from build123d import *

# Parameters (mm, degrees)
EXTRUDE1_DEPTH     = 17.78
SKETCH4_R          = 3.175000003
SKETCH4_R_2        = 3.175000002
CUT_EXTRUDE1_DEPTH = 17.78
SKETCH6_R          = 1.5875
SKETCH6_R_2        = 1.587500002
SKETCH6_R_3        = 2.777849083
CUT_EXTRUDE3_DEPTH = 17.78
SKETCH5_W          = 17.78
SKETCH5_H          = 63.50740041
SKETCH5_H_2        = 63.507400408
CUT_EXTRUDE2_DEPTH = 5.08
SKETCH7_R          = 3.302
SKETCH7_R_2        = 3.302000002
CUT_EXTRUDE4_DEPTH = 5.08
SKETCH9_R          = 3.175
CUT_EXTRUDE5_DEPTH = 17.78


with BuildPart() as part:
    # Sketch3 → Extrude1 (new body)
    with BuildSketch(Plane.XY):
        Polygon((10806.641666666, -6342.0625), (11409.891666666, -6342.0625), (11409.891666666, -5818.736838581), (11378.141666665, -5818.736838581), (11378.141666665, -5742.536838581), (10838.391666667, -5742.536838581), (10838.391666667, -5818.736838581), (10806.641666666, -5818.736838581), align=None)
    extrude(amount=-EXTRUDE1_DEPTH)

    # Sketch4 → Cut-Extrude1 (cut)
    with BuildSketch(Plane.XY):
        with Locations((11380.386730695, -5816.491774551)):
            Circle(SKETCH4_R)
        with Locations((10836.146602637, -5816.491774551)):
            Circle(SKETCH4_R_2)
    extrude(amount=-CUT_EXTRUDE1_DEPTH, mode=Mode.SUBTRACT)

    # Sketch6 → Cut-Extrude3 (cut)
    with BuildSketch(Plane.XY):
        with Locations((10851.409166666, -6294.4375)):
            Circle(SKETCH6_R)
        with Locations((10908.241666666, -6326.8225)):
            Circle(SKETCH6_R)
        with Locations((11108.266666666, -6326.8225)):
            Circle(SKETCH6_R)
        with Locations((11308.291666666, -6326.8225)):
            Circle(SKETCH6_R)
        with Locations((11365.124166666, -6294.4375)):
            Circle(SKETCH6_R)
        with Locations((11365.124166666, -6237.2875)):
            Circle(SKETCH6_R)
        with Locations((11333.691666666, -6220.099669291)):
            Circle(SKETCH6_R)
        with Locations((11365.124166666, -6180.1375)):
            Circle(SKETCH6_R)
        with Locations((11333.691666666, -6042.299669291)):
            Circle(SKETCH6_R)
        with Locations((11333.691666666, -5864.499669291)):
            Circle(SKETCH6_R)
        with Locations((11369.251666663, -5793.344238991)):
            Circle(SKETCH6_R_2)
        with Locations((11369.251666663, -5755.236838581)):
            Circle(SKETCH6_R_2)
        with Locations((10847.281666666, -5755.236838581)):
            Circle(SKETCH6_R)
        with Locations((10847.281666666, -5793.344238991)):
            Circle(SKETCH6_R)
        with Locations((10882.841666666, -6042.299669291)):
            Circle(SKETCH6_R_3)
        with Locations((10851.409166666, -6180.1375)):
            Circle(SKETCH6_R)
        with Locations((10882.841666666, -6220.099669291)):
            Circle(SKETCH6_R)
        with Locations((10851.409166666, -6237.2875)):
            Circle(SKETCH6_R)
        with Locations((10882.841666666, -5864.499669291)):
            Circle(SKETCH6_R)
    extrude(amount=-CUT_EXTRUDE3_DEPTH, mode=Mode.SUBTRACT)

    # Sketch5 → Cut-Extrude2 (cut)
    with BuildSketch(Plane.XY):
        Polygon((11108.266666666, -6317.9325), (10806.641666666, -6317.9325), (10806.641666666, -6335.7125), (11409.891666666, -6335.7125), (11409.891666666, -6317.9325), align=None)
        with Locations((10847.281666667, -5774.290538786)):
            Rectangle(SKETCH5_W, SKETCH5_H)
        with Locations((11369.251666665, -5774.290538785)):
            Rectangle(SKETCH5_W, SKETCH5_H_2)
    extrude(amount=-CUT_EXTRUDE2_DEPTH, mode=Mode.SUBTRACT)

    # Sketch7 → Cut-Extrude4 (cut)
    with BuildSketch(Plane.XY):
        with Locations((10853.926602637, -5803.79917496)):
            Circle(SKETCH7_R)
        with Locations((11362.606730695, -5803.799174959)):
            Circle(SKETCH7_R_2)
    extrude(amount=-CUT_EXTRUDE4_DEPTH, mode=Mode.SUBTRACT)

    # Sketch9 → Cut-Extrude5 (cut)
    with BuildSketch(Plane.XY):
        with Locations((10914.541654066, -5760.644320781)):
            Circle(SKETCH9_R)
        with Locations((10971.741666666, -5760.644320781)):
            Circle(SKETCH9_R)
        with Locations((11244.741654066, -5760.644320781)):
            Circle(SKETCH9_R)
        with Locations((11301.941666666, -5760.644320781)):
            Circle(SKETCH9_R)
    extrude(amount=-CUT_EXTRUDE5_DEPTH, mode=Mode.SUBTRACT)


solid = part.part
The listing builds one solid part. Answer for the finished solid, in the listing's coordinates (mm). A direction names the side the tool comes from. Coordinates: 2 decimals unless noted, no trailing zeros. Write each loop counter-clockwise with the first axis right and the second up, starting at its lowest first coordinate (ties: lowest second). Pieces come first, ordered by that corner, then holes. Notation, with made-up numbers: M 45,39.5 L 76,39.5 A26 ccw 76,66.5 Z; hole C 52.25,-7 d1. An arc over 180 degrees is marked long. Write each question's results on one line, items separated by ' | '.
Item 1: Which of the six approach directions +Z, -Z, +X, -X, +Y, -Y give full straight-line access (tool end or side, diameter ignored) to faces 1 (the face through (11396, -5818.737, -9)), 2 (the face through (11104, -6038, -17.78)), 3 (the face through (10820, -5818.737, -9))?
Answer below:
face 1: +Z, -Z, +X, +Y | face 2: -Z, +X, -X, +Y, -Y | face 3: +Z, -Z, -X, +Y
Item 2: Consider probe 1 along Y at (x, z) = (10983.5, -1.5); probe 2 along X at (y, z) = (-5807, -13.75); probe 3 along X at (y, z) = (-5778.5, -3.75). Determine where each line is inside the solid, lowest interval first. Write a range as [from, to].
Answer below:
probe 1: [-6342.06, -6335.71], [-6317.93, -5742.54] | probe 2: [10838.39, 11378.14] | probe 3: [10856.17, 11360.36]
Item 3: For a pull along Y with two mould halves and no side action, classify faces 4 (the face through (11112, -5742.537, -9)), 5 (the face through (11378.142, -5779, -11)), 6 (the face through (11104, -6327, -5.08)), 7 (the face through (11104, -6342.062, -9)) as released by +Y, released by -Y, zero draft, split by the parting line, or undercut.
Answer below:
face 4: released by +Y | face 5: zero draft | face 6: undercut | face 7: released by -Y
Item 4: Given P1, Ø3.5, axis at x = 10847.28, y = -5755.24, coming from the +Z side, flat-ended and moving along its own axis, determine where the tip first touches the part or whether it passes through.
Answer below:
P1: z = -5.08
Item 5: The part is cut by section A-A on y = -5778.5. Determine the outline of the cut face in (x, z), and give its area (3 significant figures).
Answer below:
outline: M 10838.39,-17.78 L 11378.14,-17.78 L 11378.14,-5.08 L 11360.36,-5.08 L 11360.36,0 L 10856.17,0 L 10856.17,-5.08 L 10838.39,-5.08 Z | area: 9,420 mm2
